```python
from build123d import *

# Parameters (mm, degrees)
BASE_EXTRUDE_DEPTH = 3


with BuildPart() as part:
    # Sketch1 → Base-Extrude (new body)
    with BuildSketch(Plane.XY):
        with BuildLine():
            Line((171.192957442, -40.665135082), (172.870030556, -22.31508098))
            ThreePointArc((172.870030556, -22.31508098), (175.563665965, -16.636900634), (175.142919492, -10.366304477))
            Line((175.142919492, -10.366304477), (168.744811214, -14.64960541))
            Line((168.744811214, -14.64960541), (167.075886495, -12.156677356))
            Line((167.075886495, -12.156677356), (173.841852345, -7.62710915))
            Line((173.841852345, -7.62710915), (171.850357265, -3.949661926))
            Line((171.850357265, -3.949661926), (156.57808296, -14.242043783))
            ThreePointArc((156.57808296, -14.242043783), (160.301341172, -18.851655885), (165.14064427, -22.271059484))
            Line((165.14064427, -22.271059484), (155.118780374, -33.49392187))
            Line((155.118780374, -33.49392187), (162.266864396, -33.140436707))
            Line((162.266864396, -33.140436707), (162.415219603, -36.140436707))
            Line((162.415219603, -36.140436707), (155.359396637, -36.4893594))
            Line((155.359396637, -36.4893594), (155.295598836, -41.193899126))
            Line((155.295598836, -41.193899126), (171.192957442, -40.665135082))
        make_face()
    extrude(amount=BASE_EXTRUDE_DEPTH)


solid = part.part
```
For this review, take the finished solid that the model builds, in its own axes (mm). A direction names the side the tool comes from. Round coordinates to 2 decimals unless told otherwise and drop trailing zeros. Write each loop counter-clockwise with the first axis right and the second up, starting at its lowest first coordinate (ties: lowest second). Pieces come first, ordered by that corner, then holes. Notation, with made-up numbers: (28, 20.25) -> (53, 20.25) arc R27 ccw to (53, 37.25) -> close; hole circle Ø10 at (22.5, -12.5). An arc over 180 degrees is marked (long way). One line per question, with ' | ' between items. Start each with the question number.
(1) Add section C-C, the plane x = 158.75. Write out the cut boundary in (y, z).
(2) Mouldability with a two-part tool opening along Y and no side actions: class faces 4 (the face through (160.2, -27.804, 1.479)), 5 (the face through (175.547, -16.724, 1.479)), 6 (the face through (164.321, -9.024, 1.479)) as released by +Y, released by -Y, zero draft, split by the parting line, or undercut.
(3) Tool access review of faces 1 (the face through (167.92, -13.42, 1.48)), 2 (the face through (172.86, -5.81, 1.48)), 3 (the face through (158.937, -36.312, 1.479)): name each direction out of +Z, -Z, +X, -X, +Y, -Y from which nothing blocks a thin tool from reaching the whole face with its end or side.
(4) Add section A-A, the plane x = 164.25. Write out the cut boundary in (y, z).
(5) For line 1 along Y through (x, z) = (167.5, 1.2); line 2 along Y through (x, z) = (168.5, 1.6); line 3 along Y through (x, z) = (161.75, 1.35), list the stretches that pass through material, from the lowest coordinate up. Write a range as from..to.
(6) Add section B-B, the plane z = 1.2. Write out the cut boundary in (x, y).
(7) Add section D-D, the plane y = -25. Write out the cut boundary in (x, z).
Answer list:
1) outline: (-41.08, 0) -> (-36.32, 0) -> (-36.32, 3) -> (-41.08, 3) -> close; (-33.31, 0) -> (-29.43, 0) -> (-29.43, 3) -> (-33.31, 3) -> close; (-17.24, 0) -> (-12.78, 0) -> (-12.78, 3) -> (-17.24, 3) -> close
2) face 4: undercut | face 5: split by the parting line | face 6: released by +Y
3) face 1: +Z, -Z | face 2: +Z, -Z, +X, +Y | face 3: +Z, -Z, -X
4) outline: (-40.9, 0) -> (-23.27, 0) -> (-23.27, 3) -> (-40.9, 3) -> close; (-21.78, 0) -> (-9.07, 0) -> (-9.07, 3) -> (-21.78, 3) -> close
5) line 1: -40.79..-12.79, -11.87..-6.88 | line 2: -40.75..-14.28, -11.2..-6.21 | line 3: -40.98..-36.17, -33.17..-26.07, -20.09..-10.76
6) outline: (155.12, -33.49) -> (162.27, -33.14) -> (162.42, -36.14) -> (155.36, -36.49) -> (155.3, -41.19) -> (171.19, -40.67) -> (172.87, -22.32) arc R12.46 ccw to (175.14, -10.37) -> (168.74, -14.65) -> (167.08, -12.16) -> (173.84, -7.63) -> (171.85, -3.95) -> (156.58, -14.24) arc R21.52 ccw to (165.14, -22.27) -> close
7) outline: (162.7, 0) -> (172.62, 0) -> (172.62, 3) -> (162.7, 3) -> close
